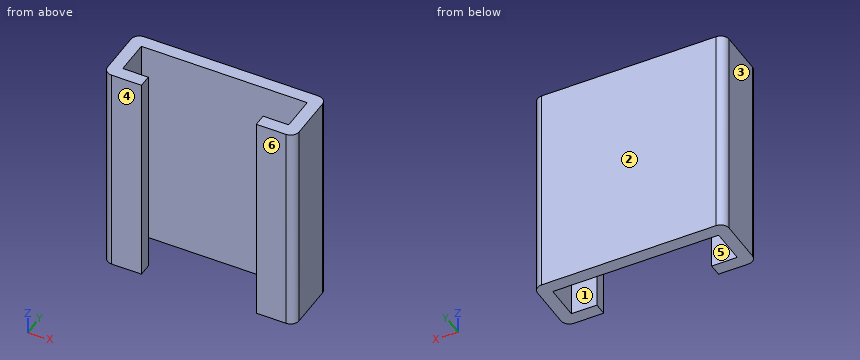
```python
from build123d import *

# Parameters (mm, degrees)
F1_DEPTH = 25.4
F2_R     = 1
F3_R     = 1


with BuildPart() as f1:
    # F0 (on Top) → F1 (new body)
    with BuildSketch(Plane.XY):
        Polygon((-9.75, 0), (0, 0), (0, 1.5), (-11.25, 1.5), (-11.25, -5.6), (-6.75, -5.6), (-6.75, -4.1), (-9.75, -4.1), align=None)
        Polygon((0, 1.5), (0, 0), (9.75, 0), (9.75, -4.1), (6.75, -4.1), (6.75, -5.6), (11.25, -5.6), (11.25, 1.5), align=None)
    extrude(amount=F1_DEPTH)

    # F2
    f2_edges = [f1.edges().sort_by_distance(p)[0] for p in [
        (-11.25, 1.5, 12.7),
        (11.25, 1.5, 12.7),
    ]]
    fillet(f2_edges, radius=F2_R)

    # F3
    f3_edges = [f1.edges().sort_by_distance(p)[0] for p in [
        (-11.25, -5.6, 12.7),
        (11.25, -5.6, 12.7),
    ]]
    fillet(f3_edges, radius=F3_R)


solid = f1.part
```
Can you work these out from the model? Positions are in its coordinate system, mm. Face numbers are marked on the shaded views. A direction names the side the tool comes from. Coordinates: 2 decimals unless noted, no trailing zeros. Loops run counter-clockwise (first coordinate to the right, second up) from the corner with the lowest first, then second, coordinate; pieces in that order, holes last. Notation, with made-up numbers: (79.25, -11) -> (86.25, -11) arc R21 cw to (86.25, 10) -> close; hole circle Ø1 at (-20.75, 54). An arc over 180 degrees is marked (long way). Put each result on its own line as item: value. Start each with the question number.
Q1. I'm going to push flat-ended pins straight in: P1, Ø4, axis at x = 2.5, y = -0.5, coming from the -Z side; P2, Ø1, axis at x = -5.5, y = -1, coming from the -Z side. Where does each tip first touch, or does it pass through?
Q2. I want a section at B-B (y = -1.75). Write out the boundary of the cut face in (x, z).
Q3. I want a section at A-A (x = 7.75). Write out the boundary of the cut face in (y, z).
Q4. Thinking about a two-plate mould opening in Y: for the marked faces 1, 2, 3 and 4, which applies, pulls with the +Y half, pulls with the -Y half, needs draft (parallel to the pull), parting line crosses it, or undercut?
Q5. I want a section at C-C (z = 8). Write out the boundary of the cut face in (x, y).
Q6. I want a section at D-D (x = 2.5). Write out the boundary of the cut face in (y, z).
Q7. For the marked faces 5 and 6, which set-ups out of +Z, -Z, +X, -X, +Y, -Y let a thin tool reach every point of the face, with its end or its side?
Q8. If I drill on line 1 (X direction, y = -2, z = 11.75); line 2 (X direction, y = -4.5, z = 15.25); line 3 (Y direction, x = -7.25, z = 14), over which ranges is the centre line in solid material (lowest first)? Write a range as [from, to].
Taken from the geometry:
1. P1: stops at z = 0
1. P2: passes through
2. outline: (-11.25, 0) -> (-9.75, 0) -> (-9.75, 25.4) -> (-11.25, 25.4) -> close; (9.75, 0) -> (11.25, 0) -> (11.25, 25.4) -> (9.75, 25.4) -> close
3. outline: (-5.6, 0) -> (-4.1, 0) -> (-4.1, 25.4) -> (-5.6, 25.4) -> close; (0, 0) -> (1.5, 0) -> (1.5, 25.4) -> (0, 25.4) -> close
4. face 1: undercut
4. face 2: pulls with the +Y half
4. face 3: needs draft
4. face 4: pulls with the -Y half
5. outline: (-11.25, -4.6) arc R1 ccw to (-10.25, -5.6) -> (-6.75, -5.6) -> (-6.75, -4.1) -> (-9.75, -4.1) -> (-9.75, 0) -> (9.75, 0) -> (9.75, -4.1) -> (6.75, -4.1) -> (6.75, -5.6) -> (10.25, -5.6) arc R1 ccw to (11.25, -4.6) -> (11.25, 0.5) arc R1 ccw to (10.25, 1.5) -> (-10.25, 1.5) arc R1 ccw to (-11.25, 0.5) -> close
6. outline: (0, 0) -> (1.5, 0) -> (1.5, 25.4) -> (0, 25.4) -> close
7. face 5: +Z, -Z
7. face 6: +Z, -Z, +X, -X, -Y
8. line 1: x = [-11.25, -9.75], [9.75, 11.25]
8. line 2: x = [-11.25, -6.75], [6.75, 11.25]
8. line 3: y = [-5.6, -4.1], [0, 1.5]
